from build123d import *

# Parameters (mm, degrees)
SKETCH1_R           = 11
SKETCH1_R_2         = 1.25
SKETCH1_R_3         = 5
BOSS_EXTRUDE7_DEPTH = 5


with BuildPart() as part:
    # Sketch1 → Boss-Extrude7 (new body)
    with BuildSketch(Plane.XY):
        with BuildLine():
            Line((-16.905, 47.876904679), (-1.9, 47.876904679))
            ThreePointArc((-1.9, 47.876904679), (18.1, 67.876904679), (38.1, 47.876904679))
            Line((38.1, 47.876904679), (53.095, 47.876904679))
            Line((53.095, 47.876904679), (53.095, -21.5))
            Line((53.095, -21.5), (53.095, -31.5))
            Line((53.095, -31.5), (33.095, -31.5))
            Line((33.095, -31.5), (33.095, -21.5))
            Line((33.095, -21.5), (3.095, -21.5))
            Line((3.095, -21.5), (3.095, -31.5))
            Line((3.095, -31.5), (-16.905, -31.5))
            Line((-16.905, -31.5), (-16.905, -21.5))
            Line((-16.905, -21.5), (-16.905, 47.876904679))
        make_face()
        with Locations((18.1, 47.876904679)):
            Circle(SKETCH1_R, mode=Mode.SUBTRACT)
        with Locations((46.095, 0)):
            Circle(SKETCH1_R_2, mode=Mode.SUBTRACT)
        with Locations((36.2, 0)):
            Circle(SKETCH1_R_3, mode=Mode.SUBTRACT)
        with Locations((26.305, 0)):
            Circle(SKETCH1_R_2, mode=Mode.SUBTRACT)
        with Locations(Location((-9.901900695, 0.004035702, 0), (0, 0, 180))):
            Circle(SKETCH1_R_2, mode=Mode.SUBTRACT)
        with Locations(Location((9.888099099, 0.001183168, 0), (0, 0, 180))):
            Circle(SKETCH1_R_2, mode=Mode.SUBTRACT)
        with Locations(Location((-0.006900798, 0.002609435, 0), (0, 0, 180))):
            Circle(SKETCH1_R_3, mode=Mode.SUBTRACT)
    extrude(amount=BOSS_EXTRUDE7_DEPTH)


solid = part.part
Read the model definition and answer for the solid it produces. Units are mm, in the model's axes. A direction names the side the tool comes from. Round coordinates to 2 decimals unless told otherwise and drop trailing zeros. Write each loop counter-clockwise with the first axis right and the second up, starting at its lowest first coordinate (ties: lowest second). Pieces come first, ordered by that corner, then holes.
Q1. Find section C-C on x = 43. Determine the outline of the cut face in (y, z), and give its area (3 significant figures).
Values:
outline: (-31.5, 0) - (47.88, 0) - (47.88, 5) - (-31.5, 5) - close
area: 397 mm2
Q2. Find section A-A on x = 18.1. Determine the outline of the cut face in (y, z).
Values:
outline: (-21.5, 0) - (36.88, 0) - (36.88, 5) - (-21.5, 5) - close; (58.88, 0) - (67.88, 0) - (67.88, 5) - (58.88, 5) - close
Q3. Find section B-B on z = 2.1. Determine the outline of the cut face in (x, y) (3 decimals).
Values:
outline: (-16.905, -31.5) - (3.095, -31.5) - (3.095, -21.5) - (33.095, -21.5) - (33.095, -31.5) - (53.095, -31.5) - (53.095, 47.877) - (38.1, 47.877) arc R20 ccw to (-1.9, 47.877) - (-16.905, 47.877) - close; hole circle Ø2.5 at (-9.902, 0.004); hole circle Ø10 at (-0.007, 0.003); hole circle Ø22 at (18.1, 47.877); hole circle Ø2.5 at (9.888, 0.001); hole circle Ø2.5 at (26.305, 0); hole circle Ø10 at (36.2, 0); hole circle Ø2.5 at (46.095, 0)
Q4. The mould has two halves that part along X. Classify faces 1 (the face through (3.961, 3.045, 2.465)), 2 (the face through (17.66, 67.872, 2.465)), 3 (the face through (19, 8, 5)): released by +X, released by -X, zero draft, split by the parting line, or undercut.
Values:
face 1: undercut
face 2: split by the parting line
face 3: zero draft
Q5. Find section D-D on x = 36. Determine the outline of the cut face in (y, z), and give its area (3 significant figures).
Values:
outline: (-31.5, 0) - (-5, 0) - (-5, 5) - (-31.5, 5) - close; (5, 0) - (56.8, 0) - (56.8, 5) - (5, 5) - close
area: 392 mm2
Q6. A flat-ended cylindrical pin translates along its axis: P1, Ø1.5, axis at x = 46.5, z = 2.5, coming from the +Y side. Find the tip coordinate at first contact, or state that the pin passes through.
Values:
P1: stops at y = 47.88
Q7. Straight lines are drawn through the part: line 1 (Y direction, x = 10, z = 0.75); line 2 (Y direction, x = 18.1, z = 1.9); line 3 (X direction, y = -22.5, z = 2.1) (3 decimals). For each, find the intervals that lie inside material, in ascending order.
Values:
line 1: y = -21.5 to -1.24, 1.25 to 40.43, 55.32 to 66.16
line 2: y = -21.5 to 36.88, 58.88 to 67.88
line 3: x = -16.905 to 3.095, 33.095 to 53.095
Q8. A tool of negligible diameter and unlimited length cuts with its end or side. For faces 4 (the face through (-7, -31.5, 2)), 5 (the face through (-16.905, 8, 2)), 6 (the face through (45, 47.877, 2)), 7 (the face through (-10, 47.877, 2)), 8 (the face through (3.095, -26, 2)), from which of +Z, -Z, +X, -X, +Y, -Y can it reach the whole face along a straight path? Write none if from no direction.
Values:
face 4: +Z, -Z, +X, -X, -Y
face 5: +Z, -Z, -X, +Y, -Y
face 6: +Z, -Z, +X, +Y
face 7: +Z, -Z, -X, +Y
face 8: +Z, -Z, -Y
